For this review, use the dimensioned drawing (mm, ordinates from the lowest corner) and the shaded views. Give positions to 0.01 mm unless a question says otherwise; leave off trailing zeros. Write each loop counter-clockwise with the first axis right and the second up, starting at its lowest first coordinate (ties: lowest second). Pieces come first, ordered by that corner, then holes. Notation, with made-up numbers: M 31.25,-25.75 L 89.25,-25.75 A15 cw 89.25,-13.75 Z; hole C 35,13 d10. An arc over 180 degrees is marked long. Answer in a Markdown table with one row per item.
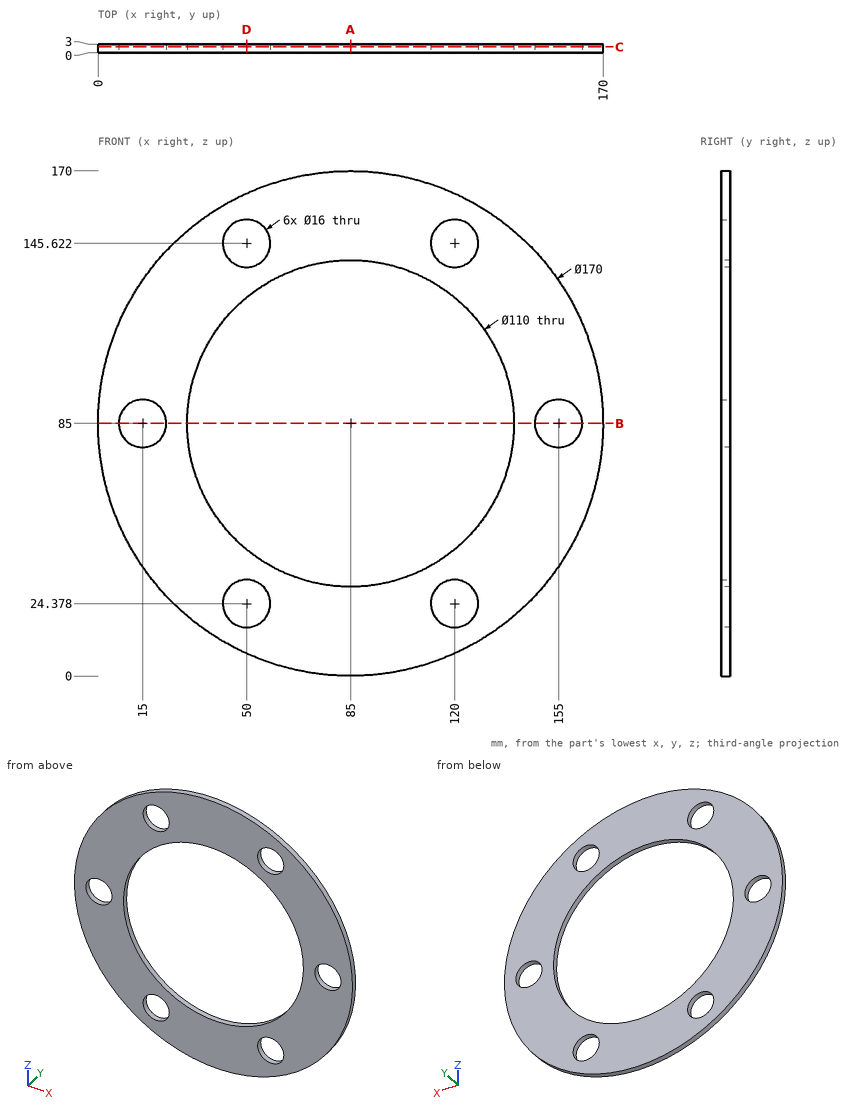
1) Add section A-A (x = 85). Write out the cut boundary in (y, z), and give its area (3 significant figures).
Geometry says:
| item | result |
|---|---|
| outline | M 0,0 L 3,0 L 3,30 L 0,30 Z; M 0,140 L 3,140 L 3,170 L 0,170 Z |
| area | 180 mm^2 |
2) Add section D-D (x = 50). Write out the cut boundary in (y, z), and give its area (3 significant figures).
Geometry says:
| item | result |
|---|---|
| outline | M 0,7.54 L 3,7.54 L 3,16.38 L 0,16.38 Z; M 0,32.38 L 3,32.38 L 3,42.57 L 0,42.57 Z; M 0,127.43 L 3,127.43 L 3,137.62 L 0,137.62 Z; M 0,153.62 L 3,153.62 L 3,162.46 L 0,162.46 Z |
| area | 114 mm^2 |
3) To check wall thickness, follow probe 1 along X at (y, z) = (1.15, 85); probe 2 along Z at (x, y) = (120, 1.2); probe 3 along X at (y, z) = (2.2, 21). State the ranges of each line that lie inside material, in increasing order. Write a range as [from, to].
Geometry says:
| item | result |
|---|---|
| probe 1 | [0, 7], [23, 30], [140, 147], [163, 170] |
| probe 2 | [7.54, 16.38], [32.38, 42.57], [127.43, 137.62], [153.62, 162.46] |
| probe 3 | [29.06, 42.75], [57.25, 112.75], [127.25, 140.94] |
4) Insertion check: P1, Ø14.5, axis at x = 15, z = 85, coming from the -Y side. The pin has a flat end and moves straight along its axis. Give the tip position at first contact, or say it passes through.
Geometry says:
| item | result |
|---|---|
| P1 | through |
5) Add section C-C (y = 2). Write out the cut boundary in (x, z), and give its area (3 significant figures).
Geometry says:
| item | result |
|---|---|
| outline | C 85,85 d170; hole C 15,85 d16; hole C 85,85 d110; hole C 50,24.38 d16; hole C 50,145.62 d16; hole C 120,24.38 d16; hole C 120,145.62 d16; hole C 155,85 d16 |
| area | 12,000 mm^2 |
6) Add section B-B (z = 85). Write out the cut boundary in (x, y), and give its area (3 significant figures).
Geometry says:
| item | result |
|---|---|
| outline | M 0,0 L 7,0 L 7,3 L 0,3 Z; M 23,0 L 30,0 L 30,3 L 23,3 Z; M 140,0 L 147,0 L 147,3 L 140,3 Z; M 163,0 L 170,0 L 170,3 L 163,3 Z |
| area | 84.0 mm^2 |
